```python
from build123d import *

# Parameters (mm, degrees)
SKETCH_1_W               = 30
SKETCH_1_H               = 40
SKETCH_1_W_2             = 27
SKETCH_1_H_2             = 36
EXTRUDE_1_DEPTH          = 90
CUT_EXTRUDE_1_REACH      = 98.954
SKETCH_2_R               = 1.6
CUT_EXTRUDE_2_DEPTH      = 99.838251704
CUT_EXTRUDE_2_DEPTH_BACK = 99.838251704
SKETCH_3_R               = 1.6


with BuildPart() as part:
    # 草图1 → 凸台-拉伸1 (new body)
    with BuildSketch(Plane(origin=(0, 0, 0), x_dir=(1, 0, 0), z_dir=(0, 1, 0))):
        Rectangle(SKETCH_1_W, SKETCH_1_H)
        Rectangle(SKETCH_1_W_2, SKETCH_1_H_2, mode=Mode.SUBTRACT)
    extrude(amount=EXTRUDE_1_DEPTH)

    # 草图2 → 切除-拉伸1 (cut, up to next)
    with BuildSketch(Plane.ZY.offset(15), mode=Mode.PRIVATE) as cut_extrude_1_sk1:
        with Locations((7.5, 78)):
            Circle(SKETCH_2_R)
    cut_extrude_1_tool1 = extrude(cut_extrude_1_sk1.sketch, amount=-CUT_EXTRUDE_1_REACH, mode=Mode.PRIVATE) & part.part
    # 草图2 → 切除-拉伸1 (cut, up to next)
    with BuildSketch(Plane.ZY.offset(15), mode=Mode.PRIVATE) as cut_extrude_1_sk2:
        with Locations((-7.5, 78)):
            Circle(SKETCH_2_R)
    cut_extrude_1_tool2 = extrude(cut_extrude_1_sk2.sketch, amount=-CUT_EXTRUDE_1_REACH, mode=Mode.PRIVATE) & part.part
    # 草图2 → 切除-拉伸1 (cut, up to next)
    with BuildSketch(Plane.ZY.offset(15), mode=Mode.PRIVATE) as cut_extrude_1_sk3:
        with Locations((-7.5, 62)):
            Circle(SKETCH_2_R)
    cut_extrude_1_tool3 = extrude(cut_extrude_1_sk3.sketch, amount=-CUT_EXTRUDE_1_REACH, mode=Mode.PRIVATE) & part.part
    # 草图2 → 切除-拉伸1 (cut, up to next)
    with BuildSketch(Plane.ZY.offset(15), mode=Mode.PRIVATE) as cut_extrude_1_sk4:
        with Locations((7.5, 62)):
            Circle(SKETCH_2_R)
    cut_extrude_1_tool4 = extrude(cut_extrude_1_sk4.sketch, amount=-CUT_EXTRUDE_1_REACH, mode=Mode.PRIVATE) & part.part
    # 草图2 → 切除-拉伸1 (cut, up to next)
    with BuildSketch(Plane.ZY.offset(15), mode=Mode.PRIVATE) as cut_extrude_1_sk5:
        with Locations((7.5, 28)):
            Circle(SKETCH_2_R)
    cut_extrude_1_tool5 = extrude(cut_extrude_1_sk5.sketch, amount=-CUT_EXTRUDE_1_REACH, mode=Mode.PRIVATE) & part.part
    # 草图2 → 切除-拉伸1 (cut, up to next)
    with BuildSketch(Plane.ZY.offset(15), mode=Mode.PRIVATE) as cut_extrude_1_sk6:
        with Locations((7.5, 12)):
            Circle(SKETCH_2_R)
    cut_extrude_1_tool6 = extrude(cut_extrude_1_sk6.sketch, amount=-CUT_EXTRUDE_1_REACH, mode=Mode.PRIVATE) & part.part
    # 草图2 → 切除-拉伸1 (cut, up to next)
    with BuildSketch(Plane.ZY.offset(15), mode=Mode.PRIVATE) as cut_extrude_1_sk7:
        with Locations((-7.5, 28)):
            Circle(SKETCH_2_R)
    cut_extrude_1_tool7 = extrude(cut_extrude_1_sk7.sketch, amount=-CUT_EXTRUDE_1_REACH, mode=Mode.PRIVATE) & part.part
    # 草图2 → 切除-拉伸1 (cut, up to next)
    with BuildSketch(Plane.ZY.offset(15), mode=Mode.PRIVATE) as cut_extrude_1_sk8:
        with Locations((-7.5, 12)):
            Circle(SKETCH_2_R)
    cut_extrude_1_tool8 = extrude(cut_extrude_1_sk8.sketch, amount=-CUT_EXTRUDE_1_REACH, mode=Mode.PRIVATE) & part.part
    add(cut_extrude_1_tool1.solids().sort_by_distance((-15, 78, 7.5))[0], mode=Mode.SUBTRACT)
    add(cut_extrude_1_tool2.solids().sort_by_distance((-15, 78, -7.5))[0], mode=Mode.SUBTRACT)
    add(cut_extrude_1_tool3.solids().sort_by_distance((-15, 62, -7.5))[0], mode=Mode.SUBTRACT)
    add(cut_extrude_1_tool4.solids().sort_by_distance((-15, 62, 7.5))[0], mode=Mode.SUBTRACT)
    add(cut_extrude_1_tool5.solids().sort_by_distance((-15, 28, 7.5))[0], mode=Mode.SUBTRACT)
    add(cut_extrude_1_tool6.solids().sort_by_distance((-15, 12, 7.5))[0], mode=Mode.SUBTRACT)
    add(cut_extrude_1_tool7.solids().sort_by_distance((-15, 28, -7.5))[0], mode=Mode.SUBTRACT)
    add(cut_extrude_1_tool8.solids().sort_by_distance((-15, 12, -7.5))[0], mode=Mode.SUBTRACT)

    # 草图3 → 切除-拉伸2 (cut, two sides: drawn at the far end of the back side and taken through both)
    with BuildSketch(Plane(origin=(0, 0, 18), x_dir=(-1, 0, 0), z_dir=(0, 0, -1)).offset(-CUT_EXTRUDE_2_DEPTH_BACK)):
        with Locations((0, 30)):
            Circle(SKETCH_3_R)
        with Locations((0, 15)):
            Circle(SKETCH_3_R)
        with Locations((0, 75)):
            Circle(SKETCH_3_R)
        with Locations((0, 60)):
            Circle(SKETCH_3_R)
    extrude(amount=CUT_EXTRUDE_2_DEPTH + CUT_EXTRUDE_2_DEPTH_BACK, mode=Mode.SUBTRACT)


solid = part.part
```
The listing builds one solid part. Answer for the finished solid, in the listing's coordinates (mm). A direction names the side the tool comes from. Coordinates: 2 decimals unless noted, no trailing zeros. Write each loop counter-clockwise with the first axis right and the second up, starting at its lowest first coordinate (ties: lowest second). Pieces come first, ordered by that corner, then holes.
Q1. Find the intervals of material crossed by line 1 along Y through (x, z) = (0, -19.5); line 2 along X through (y, z) = (75, 19.5); line 3 along X through (y, z) = (12, 10), in increasing order.
Returned:
line 1: y = 0 to 13.4, 16.6 to 28.4, 31.6 to 58.4, 61.6 to 73.4, 76.6 to 90
line 2: x = -15 to -1.6, 1.6 to 15
line 3: x = -15 to -13.5, 13.5 to 15
Q2. The mould has two halves that part along Z. Classify faces 1 (the cylindrical face through (0.208, 76.586, 19.014)), 2 (the flat face through (0, 44, 20)), 3 (the flat face through (0, 44, 18)), 4 (the flat face through (0, 44, -20)): released by +Z, released by -Z, zero draft, split by the parting line, or undercut.
Returned:
face 1: zero draft
face 2: released by +Z
face 3: undercut
face 4: released by -Z
Q3. Section A-A, the plane y = 12 is taken. Write down the section's boundary in (x, z).
Returned:
outline: (-15, -20) - (15, -20) - (15, 20) - (-15, 20) - (-15, 9.1) - (-13.5, 9.1) - (-13.5, 18) - (13.5, 18) - (13.5, -18) - (-13.5, -18) - (-13.5, -9.1) - (-15, -9.1) - close; (-15, -5.9) - (-13.5, -5.9) - (-13.5, 5.9) - (-15, 5.9) - close
Q4. Section C-C, the plane x = -10.25 is taken. Write down the section's boundary in (y, z).
Returned:
outline: (0, -20) - (90, -20) - (90, -18) - (0, -18) - close; (0, 18) - (90, 18) - (90, 20) - (0, 20) - close
Q5. Section B-B, the plane z = -17 is taken. Write down the section's boundary in (x, y), then the cut area to 3 significant figures.
Returned:
outline: (-15, 0) - (-13.5, 0) - (-13.5, 90) - (-15, 90) - close; (13.5, 0) - (15, 0) - (15, 90) - (13.5, 90) - close
area: 270 mm2
Q6. Which of the six approach directions +Z, -Z, +X, -X, +Y, -Y give full straight-line access (tool end or side, diameter ignored) to faces 5 (the cylindrical face through (-14.26, 63.586, -7.708)), 6 (the flat face through (13.5, 44, 0)), 7 (the cylindrical face through (0.208, 16.586, 19.014))?
Returned:
face 5: -X
face 6: +Y, -Y
face 7: +Z, -Z
Q7. Section D-D, the plane z = -7.5 is taken. Write down the section's boundary in (x, y), then the cut area to 3 significant figures.
Returned:
outline: (-15, 0) - (-13.5, 0) - (-13.5, 10.4) - (-15, 10.4) - close; (-15, 13.6) - (-13.5, 13.6) - (-13.5, 26.4) - (-15, 26.4) - close; (-15, 29.6) - (-13.5, 29.6) - (-13.5, 60.4) - (-15, 60.4) - close; (-15, 63.6) - (-13.5, 63.6) - (-13.5, 76.4) - (-15, 76.4) - close; (-15, 79.6) - (-13.5, 79.6) - (-13.5, 90) - (-15, 90) - close; (13.5, 0) - (15, 0) - (15, 90) - (13.5, 90) - close
area: 251 mm2
Q8. Given P1, Ø1.9, axis at y = 28, z = 7.5, coming from the -X side; P2, Ø2.5, axis at x = 0, y = 75, coming from the +Z side (3 decimals), each flat-ended and moving along its own axis, determine where each tip first touches the part or whether it passes through.
Returned:
P1: stops at x = 13.5
P2: passes through
